from build123d import *

# Parameters (mm, degrees)
BOSS_EXTRUDE1_DEPTH = 15
SKETCH3_R           = 2.5
SKETCH3_R_2         = 12.5
CUT_EXTRUDE1_DEPTH  = 100.686506887


with BuildPart() as part:
    # Sketch1 → Boss-Extrude1 (new body)
    with BuildSketch(Plane(origin=(0, 0, 0), x_dir=(1, 0, 0), z_dir=(0, 1, 0))):
        Polygon((0, 0), (29, 79.676845164), (58, 0), align=None)
        Polygon((0, 0), (58, 0), (29, -79.676845164), align=None)
    extrude(amount=BOSS_EXTRUDE1_DEPTH)

    # Sketch3 → Cut-Extrude1 (cut, through all)
    with BuildSketch(Plane.XZ):
        with Locations(Location((28.720595315, 59.676845164, 0), (0, 0, 270))):
            Circle(SKETCH3_R)
        with Locations(Location((28.971190629, 39.676845164, 0), (0, 0, 270))):
            Circle(SKETCH3_R_2)
        with Locations(Location((28.971190629, 19.676845164, 0), (0, 0, 270))):
            Circle(SKETCH3_R)
        with Locations(Location((28.720595315, -59.676845164, 0), (0, 0, 90))):
            Circle(SKETCH3_R)
        with Locations(Location((28.971190629, -19.676845164, 0), (0, 0, 90))):
            Circle(SKETCH3_R)
        with Locations(Location((28.971190629, -39.676845164, 0), (0, 0, 90))):
            Circle(SKETCH3_R_2)
    extrude(amount=-CUT_EXTRUDE1_DEPTH, mode=Mode.SUBTRACT)


solid = part.part
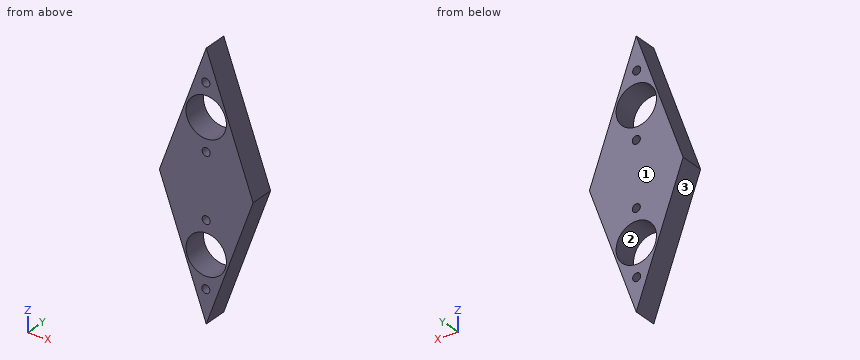
Read the model definition and answer for the solid it produces. Units are mm, in the model's axes. Face numbers are marked on the shaded views. Coordinates: 2 decimals unless noted, no trailing zeros. Order: outer loops, then holes, each group sorted by start corner. A loop starts at its lowest first (then second) coordinate and runs counter-clockwise, first axis right, second up. Notation, with made-up numbers: (63, 31.25) -> (77, 31.25) arc R11 ccw to (77, 44.25) -> close; hole circle Ø4 at (85.5, 53.25). An arc over 180 degrees is marked (long way). Answer as a JSON object with one key per item and string values.
1) A cutting plane is placed at A-A, the plane x = 22. Determine the outline of the cut face in (y, z), plus the area to 3 significant figures.
Model answer:
{"outline": "(0, -60.44) -> (15, -60.44) -> (15, -50.05) -> (0, -50.05) -> close; (0, -29.3) -> (15, -29.3) -> (15, 29.3) -> (0, 29.3) -> close; (0, 50.05) -> (15, 50.05) -> (15, 60.44) -> (0, 60.44) -> close", "area": "1,190 mm²"}
2) A cutting plane is placed at D-D, the plane z = 8. Determine the outline of the cut face in (x, y).
Model answer:
{"outline": "(2.91, 0) -> (55.09, 0) -> (55.09, 15) -> (2.91, 15) -> close"}
3) The mould has two halves that part along X. Classify the marked faces 1, 2 and 3: released by +X, released by -X, zero draft, split by the parting line, or undercut.
Model answer:
{"face 1": "zero draft", "face 2": "undercut", "face 3": "released by -X"}
4) A cutting plane is placed at C-C, the plane x = 8.5. Determine the outline of the cut face in (y, z).
Model answer:
{"outline": "(0, -23.35) -> (15, -23.35) -> (15, 23.35) -> (0, 23.35) -> close"}
5) A cutting plane is placed at B-B, the plane y = 9. Determine the outline of the cut face in (x, z).
Model answer:
{"outline": "(0, 0) -> (29, -79.68) -> (58, 0) -> (29, 79.68) -> close; hole circle Ø25 at (28.97, -39.68); hole circle Ø25 at (28.97, 39.68); hole circle Ø5 at (28.72, -59.68); hole circle Ø5 at (28.72, 59.68); hole circle Ø5 at (28.97, -19.68); hole circle Ø5 at (28.97, 19.68)"}
6) Consider line 1 along X through (y, z) = (11.5, -50); line 2 along X through (y, z) = (7.5, -37.5); line 3 along X through (y, z) = (14.25, 3). Determine where each line is inside the solid, lowest interval first. Write a range as from..to.
Model answer:
{"line 1": "x = 18.2..21.92, 36.02..39.8", "line 2": "x = 13.65..16.66, 41.28..44.35", "line 3": "x = 1.09..56.91"}
7) Each of these flat-tipped pins is pushed along its axis until it touches: pin 1 (3 mm diameter, centred on x = 28.97, z = 19.68, fed in from -Y); pin 2 (3 mm diameter, centred on y = 4, z = -41, fed in from +X); pin 3 (1.5 mm diameter, centred on y = 8, z = -49.5, fed in from -X). Where does it stop, or does it pass through?
Model answer:
{"pin 1": "passes through", "pin 2": "stops at x = 43.62", "pin 3": "stops at x = 17.74"}
